```python
from build123d import *

# Parameters (mm, degrees)
ESQUISSE1_W              = 100
ESQUISSE1_H              = 100
BOSS_EXTRU_1_DEPTH       = 25
ESQUISSE2_R              = 7.9
ESQUISSE2_R_2            = 7.95
ESQUISSE2_R_3            = 4.5
ENL_V_MAT_EXTRU_1_DEPTH  = 144.614066163
ESQUISSE3_R              = 4.3
ENL_V_MAT_EXTRU_3_DEPTH  = 10
ESQUISSE4_W              = 7
ESQUISSE4_H              = 42
BOSS_EXTRU_2_DEPTH       = 42.3
ESQUISSE5_R              = 1.5
ENL_V_MAT_EXTRU_4_DEPTH  = 12
ESQUISSE6_W              = 40
ESQUISSE6_H              = 100
ENL_V_MAT_EXTRU_6_DEPTH  = 148.61195751
ENL_V_MAT_EXTRU_8_DEPTH  = 7.5
ESQUISSE10_R             = 11.5
ENL_V_MAT_EXTRU_10_DEPTH = 119.314369372
ESQUISSE11_R             = 1.5
ENL_V_MAT_EXTRU_11_DEPTH = 3
ESQUISSE12_W             = 60
ESQUISSE12_H             = 23
ENL_V_MAT_EXTRU_12_DEPTH = 148.61195751
CONG_1_R                 = 2


with BuildPart() as part:
    # Esquisse1 → Boss.-Extru.1 (new body)
    with BuildSketch(Plane.XY):
        with Locations((50, 50)):
            Rectangle(ESQUISSE1_W, ESQUISSE1_H)
    extrude(amount=BOSS_EXTRU_1_DEPTH)

    # Esquisse2 → Enlèv. mat.-Extru.1 (cut, through all)
    with BuildSketch(Plane.XY):
        with Locations((61.7000009, 9.994583957)):
            Circle(ESQUISSE2_R)
        with Locations((78, 10)):
            Circle(ESQUISSE2_R_2)
        with Locations((69.845134328, 24.642259589)):
            Circle(ESQUISSE2_R_3)
    extrude(amount=ENL_V_MAT_EXTRU_1_DEPTH, mode=Mode.SUBTRACT)

    # Esquisse3 → Enlèv. mat.-Extru.3 (cut)
    with BuildSketch(Plane(origin=(0, 0, 0), x_dir=(1, 0, 0), z_dir=(0, 1, 0))):
        with Locations(Location((48, -12.5, 0), (0, 0, 270))):
            Circle(ESQUISSE3_R)
        with Locations(Location((92, -12.5, 0), (0, 0, 270))):
            Circle(ESQUISSE3_R)
    extrude(amount=ENL_V_MAT_EXTRU_3_DEPTH, mode=Mode.SUBTRACT)

    # Esquisse4 → Boss.-Extru.2 (add)
    with BuildSketch(Plane.XY):
        with Locations((56.5, 56)):
            Rectangle(ESQUISSE4_W, ESQUISSE4_H)
    extrude(amount=-BOSS_EXTRU_2_DEPTH)

    # Esquisse5 → Enlèv. mat.-Extru.4 (cut)
    with BuildSketch(Plane(origin=(60, 0, 0), x_dir=(0, 0, -1), z_dir=(1, 0, 0))):
        with Locations(Location((36.65, 71.35, 0), (0, 0, 90))):
            Circle(ESQUISSE5_R)
        with Locations(Location((36.65, 40.65, 0), (0, 0, 90))):
            Circle(ESQUISSE5_R)
        with Locations(Location((5.65, 40.65, 0), (0, 0, 90))):
            Circle(ESQUISSE5_R)
        with Locations(Location((5.65, 71.35, 0), (0, 0, 90))):
            Circle(ESQUISSE5_R)
    extrude(amount=-ENL_V_MAT_EXTRU_4_DEPTH, mode=Mode.SUBTRACT)

    # Esquisse6 → Enlèv. mat.-Extru.6 (cut, through all)
    with BuildSketch(Plane.XY):
        with Locations((20, 50)):
            Rectangle(ESQUISSE6_W, ESQUISSE6_H)
    extrude(amount=ENL_V_MAT_EXTRU_6_DEPTH, mode=Mode.SUBTRACT)

    # Esquisse8 → Enlèv. mat.-Extru.8 (cut)
    with BuildSketch(Plane(origin=(0, 0, 0), x_dir=(-1, 0, 0), z_dir=(0, 0, -1))):
        Polygon((-62.690994399, 21.852704928), (-63.852239162, 29.44314918), (-71.006379091, 32.232703841), (-76.999274258, 27.43181425), (-75.838029495, 19.841369999), (-68.683889565, 17.051815338), align=None)
    extrude(amount=-ENL_V_MAT_EXTRU_8_DEPTH, mode=Mode.SUBTRACT)

    # Esquisse10 → Enlèv. mat.-Extru.10 (cut, through all)
    with BuildSketch(Plane.ZY.offset(-53)):
        with Locations((-21.15, 56.15)):
            Circle(ESQUISSE10_R)
    extrude(amount=-ENL_V_MAT_EXTRU_10_DEPTH, mode=Mode.SUBTRACT)

    # Esquisse11 → Enlèv. mat.-Extru.11 (cut)
    with BuildSketch(Plane(origin=(100, 0, 0), x_dir=(0, 0, -1), z_dir=(1, 0, 0))):
        with Locations((-15.163954836, 26)):
            Circle(ESQUISSE11_R)
        with Locations((-15.163954836, 14.75187619)):
            Circle(ESQUISSE11_R)
    extrude(amount=-ENL_V_MAT_EXTRU_11_DEPTH, mode=Mode.SUBTRACT)

    # Esquisse12 → Enlèv. mat.-Extru.12 (cut, through all)
    with BuildSketch(Plane(origin=(0, 0, 0), x_dir=(-1, 0, 0), z_dir=(0, 0, -1))):
        with Locations((-70, 88.5)):
            Rectangle(ESQUISSE12_W, ESQUISSE12_H)
    extrude(amount=-ENL_V_MAT_EXTRU_12_DEPTH, mode=Mode.SUBTRACT)

    # Congé1
    cong_1_edges = [part.edges().sort_by_distance(p)[0] for p in [
        (100, 77, 12.5),
        (40, 77, 12.5),
        (40, 0, 12.5),
        (100, 0, 12.5),
    ]]
    fillet(cong_1_edges, radius=CONG_1_R)


solid = part.part
```
The model under review builds one solid part; all positions refer to its coordinate system, in mm. A direction names the side the tool comes from. Give positions to 0.01 mm unless a question says otherwise; leave off trailing zeros. Loops run counter-clockwise (first coordinate to the right, second up) from the corner with the lowest first, then second, coordinate; pieces in that order, holes last. Notation, with made-up numbers: (60, -19) -> (105, -19) arc R23 cw to (105, -3) -> close; hole circle Ø4 at (88.25, -22). An arc over 180 degrees is marked (long way). Use CSV: the item, a comma, the result in double quotes.
1. Consider section D-D, the plane y = 71.35. Write out the cut boundary in (x, z), then the cut area to 3 significant figures.
Result:
outline,"(40, 0) -> (53, 0) -> (53, -4.15) -> (60, -4.15) -> (60, 0) -> (100, 0) -> (100, 25) -> (40, 25) -> close; (53, -42.3) -> (60, -42.3) -> (60, -38.15) -> (53, -38.15) -> close; (53, -35.15) -> (60, -35.15) -> (60, -7.15) -> (53, -7.15) -> close"
area,"1,750 mm²"
2. For P1, Ø4, axis at y = 40.65, z = -36.65, coming from the -X side; P2, Ø1.5, axis at y = 26.5, z = 15.5, coming from the +X side; P3, Ø11.5, axis at x = 69.5, y = 21.5, coming from the -Z side, all flat-tipped, find the tip position at first contact; note any pin that passes through.
Result:
P1,"stops at x = 53"
P2,"stops at x = 97"
P3,"stops at z = 0"
3. Consider section A-A, the plane x = 78. Write out the cut boundary in (y, z), then the cut area to 3 significant figures.
Result:
outline,"(0, 0) -> (2.05, 0) -> (2.05, 25) -> (0, 25) -> close; (17.95, 0) -> (77, 0) -> (77, 25) -> (17.95, 25) -> close"
area,"1,530 mm²"
4. Consider section B-B, the plane y = 56.15. Write out the cut boundary in (x, z).
Result:
outline,"(40, 0) -> (53, 0) -> (53, -9.65) -> (60, -9.65) -> (60, 0) -> (100, 0) -> (100, 25) -> (40, 25) -> close; (53, -42.3) -> (60, -42.3) -> (60, -32.65) -> (53, -32.65) -> close"
5. Machinability: for faces 1 (the face through (60, 65, -11)), 2 (the face through (56, 35, -21)), 3 (the face through (65, 25, 7.5)), which of the approach directions +Z, -Z, +X, -X, +Y, -Y give a long, thin tool a straight path to every point of the face, cutting with its end or side? Answer none if there is none.
Result:
face 1,"-Z, +X, +Y, -Y"
face 2,"-Z, +X, -X, -Y"
face 3,"-Z"
6. The part is to be moulded in two halves that separate along Z. For faces 4 (the face through (70, 77, 6)), 5 (the face through (70, 39, 0)), 6 (the face through (95.626, 4.93, 14.812)), say which applies: +Z half, -Z half, draft (parallel to the pull), parting line (faces both ways), or undercut.
Result:
face 4,"draft"
face 5,"-Z half"
face 6,"undercut"
7. To check wall thickness, follow probe 1 along Z at (x, y) = (55, 71); probe 2 along X at (y, z) = (10, 5.5); probe 3 along X at (y, z) = (7, 8). State the ranges of each line that lie inside material, in increasing order. Write a range as from..to.
Result:
probe 1,"z = -42.3..-38.11, -35.19..-7.11, -4.19..25"
probe 2,"x = 40..53.8, 69.6..70.05, 85.95..100"
probe 3,"x = 40..54.39, 69.01..70.64, 85.36..100"
8. Consider section C-C, the plane z = -21.15. Write out the cut boundary in (x, y).
Result:
outline,"(53, 35) -> (60, 35) -> (60, 44.65) -> (53, 44.65) -> close; (53, 67.65) -> (60, 67.65) -> (60, 77) -> (53, 77) -> close"
